Can you work these out from the model? Positions are in its coordinate system, mm. Face numbers are marked on the shaded views. Give positions to 0.01 mm unless a question says otherwise; leave off trailing zeros. Order: outer loops, then holes, each group sorted by start corner. A loop starts at its lowest first (then second) coordinate and runs counter-clockwise, first axis right, second up.
Item 1: If I drill on line 1 along Z through (x, y) = (12, -2.95); line 2 along X through (y, z) = (-2.4, -2.25); line 3 along X through (y, z) = (-0.3, -3.25), over which ranges is the centre line in solid material (lowest first)?
Item 2: I want a section at A-A, the plane z = -2.5. Write out the boundary of the cut face in (x, y).
Item 3: I want a section at C-C, the plane y = -0.6. Write out the boundary of the cut face in (x, z), then the cut area to 3 significant figures.
Item 4: If we mould it in two halves opening along Z, with no side actions, what happens to the marked faces 1, 2 and 3? For each: +Z half, -Z half, draft (parallel to the pull), parting line (faces both ways), or undercut.
Item 5: I want a section at B-B, the plane x = 12. Write out the boundary of the cut face in (y, z), then the cut area to 3 significant figures.
Item 6: I'm going to push a flat-ended pin straight in: pin 1 Ø4 at (x, z) = (-12, -2.5) entering from +Y. Where does the tip first touch, or does it pass through?
Item 7: I want a section at D-D, the plane x = -7. Write out the boundary of the cut face in (y, z), then the cut area to 3 significant figures.
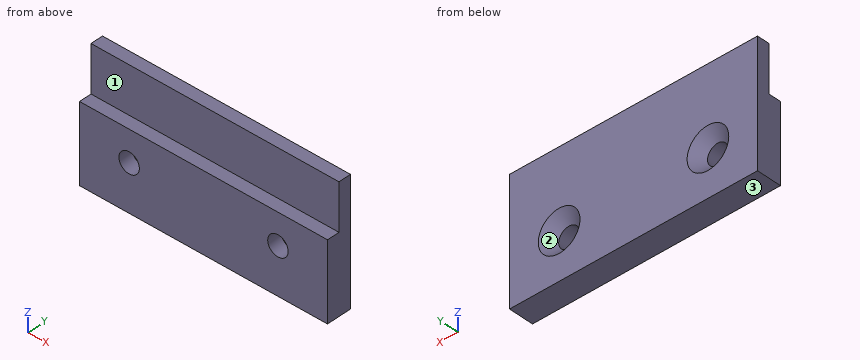
```python
from build123d import *

# Parameters (mm, degrees)
F0_W           = 40
F0_H           = 7.5
F1_DEPTH       = 2
F0_H_2         = 12.5
F2_DEPTH       = 4
F3_D           = 3.3
F3_CSINK_D     = 6.72
F3_CSINK_ANGLE = 90


with BuildPart() as f1:
    # F0 (on Front) → F1 (new body)
    with BuildSketch(Plane.XZ):
        with Locations((0, 6.25)):
            Rectangle(F0_W, F0_H)
    extrude(amount=F1_DEPTH)

    # F0 (on Front) → F2 (join)
    with BuildSketch(Plane.XZ):
        with Locations((0, -3.75)):
            Rectangle(F0_W, F0_H_2)
    extrude(amount=F2_DEPTH)

    # F3 (through all)
    with Locations(Plane(origin=(0, 0, 0), x_dir=(1, 0, 0), z_dir=(0, 1, 0))):
        with Locations((-12, 2.5), (12, 2.5)):
            CounterSinkHole(F3_D / 2, F3_CSINK_D / 2, counter_sink_angle=F3_CSINK_ANGLE)


solid = f1.part
```
Results list:
1. line 1: z = -10 to -4.15, -0.85 to 2.5
1. line 2: x = -20 to -13.63, -10.37 to 10.37, 13.63 to 20
1. line 3: x = -20 to -14.97, -9.03 to 9.03, 14.97 to 20
2. outline: (-20, -4) - (-13.65, -4) - (-13.65, -1.71) - (-15.36, 0) - (-20, 0) - close; (-10.35, -4) - (10.35, -4) - (10.35, -1.71) - (8.64, 0) - (-8.64, 0) - (-10.35, -1.71) - close; (13.65, -4) - (20, -4) - (20, 0) - (15.36, 0) - (13.65, -1.71) - close
3. outline: (-20, -10) - (20, -10) - (20, 10) - (-20, 10) - close; hole circle Ø5.52 at (-12, -2.5); hole circle Ø5.52 at (12, -2.5)
3. area: 752 mm2
4. face 1: draft
4. face 2: undercut
4. face 3: -Z half
5. outline: (-4, -10) - (0, -10) - (0, -5.86) - (-1.71, -4.15) - (-4, -4.15) - close; (-4, -0.85) - (-1.71, -0.85) - (0, 0.86) - (0, 10) - (-2, 10) - (-2, 2.5) - (-4, 2.5) - close
5. area: 48.9 mm2
6. pin 1: stops at y = -1.36
7. outline: (-4, -10) - (0, -10) - (0, 10) - (-2, 10) - (-2, 2.5) - (-4, 2.5) - close
7. area: 65.0 mm2
